Read the model definition and answer for the solid it produces. Units are mm, in the model's axes. A direction names the side the tool comes from. Give positions to 0.01 mm unless a question says otherwise; leave off trailing zeros. Write each loop counter-clockwise with the first axis right and the second up, starting at its lowest first coordinate (ties: lowest second). Pieces come first, ordered by that corner, then holes. Notation, with made-up numbers: (-16.75, 45) -> (21.25, 45) arc R7 ccw to (21.25, 52) -> close; hole circle Ø8 at (65.5, 43.5). An arc over 180 degrees is marked (long way). Use a Markdown table: item, result.
from build123d import *

# Parameters (mm, degrees)
F1_DEPTH = 12
F2_R     = 1.1
F3_DEPTH = 6.5
F4_R     = 2.5
F5_DEPTH = 25


with BuildPart() as f1:
    # F0 (on Right) → F1 (new body)
    with BuildSketch(Plane.YZ):
        Polygon((25.1, -0.075058), (-4.9, -0.075058), (-4.9, -25.075058), (0, -25.075058), (0, -10.075058), (3.1, -10.075058), (3.1, -25.075058), (25.1, -25.075058), align=None)
    extrude(amount=F1_DEPTH)

    # F2 (on face) → F3 (cut)
    with BuildSketch(Plane.YZ.offset(12)):
        Polygon((24.6, -2.396713), (8.6, -2.396713), (8.6, -22.896713), (24.6, -22.896713), (24.6, -13.396713), (28.479045, -13.396713), (28.479045, -2.396713), align=None)
        with Locations((16.6, -17.646713)):
            Circle(F2_R, mode=Mode.SUBTRACT)
        with Locations((16.6, -7.646713)):
            Circle(F2_R, mode=Mode.SUBTRACT)
    extrude(amount=-F3_DEPTH, mode=Mode.SUBTRACT)

    # F4 (on face) → F5 (cut)
    with BuildSketch(Plane(origin=(0, 8.6, 0), x_dir=(-1, 0, 0), z_dir=(0, 1, 0))):
        with Locations((-8.783709, -5.351877)):
            Circle(F4_R)
    extrude(amount=-F5_DEPTH, mode=Mode.SUBTRACT)


solid = f1.part
Item 1: Straight lines are drawn through the part: line 1 along Y through (x, z) = (8, -19.25); line 2 along Z through (x, y) = (9.5, 16.5); line 3 along Y through (x, z) = (2.75, -13.5). For each, find the intervals that lie inside material, in ascending order. Write a range as [from, to].
Return value:
| item | result |
|---|---|
| line 1 | [-4.9, 0], [3.1, 8.6], [24.6, 25.1] |
| line 2 | [-25.08, -22.9], [-18.74, -16.55], [-8.74, -6.55], [-2.4, -0.08] |
| line 3 | [-4.9, 0], [3.1, 25.1] |
Item 2: Each of these flat-tipped pins is pushed along its axis until it touches: P1, Ø4, axis at x = 8.78, z = -5.35, coming from the -Y side; P2, Ø12, axis at y = 15, z = -16, coming from the -X side; P3, Ø1, axis at y = 18.5, z = -15.5, coming from the +X side; P4, Ø0.9, axis at x = 8.5, y = 2.5, coming from the -Z side. Where does it stop, or does it pass through?
Return value:
| item | result |
|---|---|
| P1 | y = 15.54 |
| P2 | x = 0 |
| P3 | x = 5.5 |
| P4 | z = -10.08 |
Item 3: A tool of negligible diameter and unlimited length cuts with its end or side. For faces 4 (the face through (9, 16, -22.897)), 5 (the face through (6, 2, -10.075)), 6 (the face through (6.4, 1.9, -4.6)), from which of +Z, -Z, +X, -X, +Y, -Y can it reach the whole face along a straight path? Write none if from no direction.
Return value:
| item | result |
|---|---|
| face 4 | +X |
| face 5 | -Z, +X, -X |
| face 6 | -Y |
Item 4: A cutting plane is placed at C-C (x = 10). Give the vertices of the cut face in (y, z), then the cut area to 3 significant figures.
Return value:
| item | result |
|---|---|
| outline | (-4.9, -25.08) -> (0, -25.08) -> (0, -10.08) -> (3.1, -10.08) -> (3.1, -25.08) -> (25.1, -25.08) -> (25.1, -13.4) -> (24.6, -13.4) -> (24.6, -22.9) -> (8.6, -22.9) -> (8.6, -7.54) -> (-4.9, -7.54) -> close; (-4.9, -3.17) -> (8.6, -3.17) -> (8.6, -2.4) -> (25.1, -2.4) -> (25.1, -0.08) -> (-4.9, -0.08) -> close; circle Ø2.2 at (16.6, -17.65); circle Ø2.2 at (16.6, -7.65) |
| area | 319 mm^2 |
Item 5: A cutting plane is placed at D-D (x = 3.25). Give the vertices of the cut face in (y, z).
Return value:
| item | result |
|---|---|
| outline | (-4.9, -25.08) -> (0, -25.08) -> (0, -10.08) -> (3.1, -10.08) -> (3.1, -25.08) -> (25.1, -25.08) -> (25.1, -0.08) -> (-4.9, -0.08) -> close |
Item 6: A cutting plane is placed at B-B (y = 11.75). Give the vertices of the cut face in (x, z).
Return value:
| item | result |
|---|---|
| outline | (0, -25.08) -> (12, -25.08) -> (12, -22.9) -> (5.5, -22.9) -> (5.5, -2.4) -> (12, -2.4) -> (12, -0.08) -> (0, -0.08) -> close |
Item 7: A cutting plane is placed at A-A (z = -20.25). Give the vertices of the cut face in (x, y).
Return value:
| item | result |
|---|---|
| outline | (0, -4.9) -> (12, -4.9) -> (12, 0) -> (0, 0) -> close; (0, 3.1) -> (12, 3.1) -> (12, 8.6) -> (5.5, 8.6) -> (5.5, 24.6) -> (12, 24.6) -> (12, 25.1) -> (0, 25.1) -> close |
Item 8: For a pull along Y with two mould halves and no side action, classify faces 1 (the face through (12, 17, -18)), 2 (the face through (5, 25.1, -13)), 3 (the face through (8.796, 16.457, -16.556)) as +Y half, -Y half, draft (parallel to the pull), parting line (faces both ways), or undercut.
Return value:
| item | result |
|---|---|
| face 1 | draft |
| face 2 | +Y half |
| face 3 | undercut |
